Read the model definition and answer for the solid it produces. Units are mm, in the model's axes. A direction names the side the tool comes from. Coordinates: 2 decimals unless noted, no trailing zeros. Loops run counter-clockwise (first coordinate to the right, second up) from the corner with the lowest first, then second, coordinate; pieces in that order, holes last. Notation, with made-up numbers: (-12, 51) - (6, 51) arc R19 ccw to (6, 59) - close; hole circle Ø1 at (-32.75, -1). An arc over 180 degrees is marked (long way). Use one line per item in the form item = value. Start each with the question number.
1) A cutting plane is placed at D-D (y = -17.25). Give the vertices of the cut face in (x, z) (1 decimal).
2) A cutting plane is placed at B-B (x = -19.5). Give the vertices of the cut face in (y, z) (3 decimals).
3) The mould has two halves that part along Z. Classify faces 1 (the face through (3, -20.955, -34)), 2 (the face through (40.42, -14, 0)), 3 (the face through (6.616, -14, 35)), 4 (the face through (-20.493, -14.087, -34.841)): released by +Z, released by -Z, zero draft, split by the parting line, or undercut.
4) A cutting plane is placed at A-A (y = -25.5). Give the vertices of the cut face in (x, z), and give its area (3 significant figures).
5) Which of the six approach directions +Z, -Z, +X, -X, +Y, -Y give full straight-line access (tool end or side, diameter ignored) to faces 5 (the face through (-3, -7.62, -34)), 6 (the face through (20.493, -14.087, 34.841)), 7 (the face through (-6.616, -14, 35))?
6) Each of these flat-tipped pins is pushed along its axis until it touches: P1, Ø2, axis at x = 28.5, y = -17.5, coming from the -Z side; P2, Ø5.5, axis at y = -16, z = 35.5, coming from the -X side; P3, Ø5.5, axis at y = -14, z = 36, coming from the +X side; P4, Ø2, axis at x = 5, z = -37.5, coming from the +Y side. Where does it stop, or does it pass through?
7) A cutting plane is placed at C-C (z = 30.5). Give the vertices of the cut face in (x, y) (3 decimals), and give its area (3 significant figures).
8) Consider line 1 (X direction, y = -11, z = 0); line 2 (X direction, y = -23.25, z = 0); line 3 (Y direction, x = -18, z = -31) (3 decimals). Determine where each line is inside the solid, lowest interval first.
from build123d import *
from build123d import SkipClean  # not in build123d's __all__

# Parameters (mm, degrees)
F0_R     = 44.45
F1_DEPTH = 38.1
F2_R     = 50.8
F3_DEPTH = 10.16
F4_R     = 50.8
F5_DEPTH = 10.16
F7_DEPTH = 25.4
F8_SCALE = 0.75


with BuildPart() as f1:
    # F0 (on Front) → F1 (new body)
    with BuildSketch(Plane.XZ):
        Polygon((53.8927608775, 31.115), (0, 62.23), (-53.8927608775, 31.115), (-53.8927608775, -31.115), (0, -62.23), (53.8927608775, -31.115), align=None)
        Circle(F0_R, mode=Mode.SUBTRACT)
    extrude(amount=F1_DEPTH)

    # F2 (on face) → F3 (cut)
    with BuildSketch(Plane.XZ.offset(38.1)):
        Circle(F2_R)
    extrude(amount=-F3_DEPTH, mode=Mode.SUBTRACT)

    # F4 (on face) → F5 (cut)
    with BuildSketch(Plane(origin=(0, 0, 0), x_dir=(-1, 0, 0), z_dir=(0, 1, 0))):
        Circle(F4_R)
    extrude(amount=-F5_DEPTH, mode=Mode.SUBTRACT)

    # F6 (on face) → F7 (cut)
    with BuildSketch(Plane(origin=(0, -10.16, 0), x_dir=(-1, 0, 0), z_dir=(0, 1, 0))):
        with BuildLine():
            Line((7.7186614973, 43.7747046214), (8.8213274255, 50.028233853))
            ThreePointArc((8.8213274255, 50.028233853), (0, 50.8), (-8.8213274255, 50.028233853))
            Line((-8.8213274255, 50.028233853), (-7.7186614973, 43.7747046214))
            ThreePointArc((-7.7186614973, 43.7747046214), (0, 44.45), (7.7186614973, 43.7747046214))
        make_face()
        with BuildLine():
            Line((-7.7186614973, 43.7747046214), (-8.8213274255, 50.028233853))
            Line((-8.8213274255, 50.028233853), (-8.8213274255, 43.5658889781))
            ThreePointArc((-8.8213274255, 43.5658889781), (-8.2706535041, 43.6737769218), (-7.7186614973, 43.7747046214))
        make_face()
        with BuildLine():
            Line((8.8213274255, 43.5658889781), (8.8213274255, 50.028233853))
            Line((8.8213274255, 50.028233853), (7.7186614973, 43.7747046214))
            ThreePointArc((7.7186614973, 43.7747046214), (8.2706535041, 43.6737769218), (8.8213274255, 43.5658889781))
        make_face()
    with SkipClean():  # cleaning this boolean's faces spoils the solid; the shape is the same uncleaned
        extrude(amount=-F7_DEPTH, mode=Mode.SUBTRACT)


with BuildPart() as f1_1:
    # F8: moved
    add(f1.part.scale(F8_SCALE), clean=False)


solid = f1_1.part
Found:
q1.outline = (-40.4, -23.3) - (0, -46.7) - (40.4, -23.3) - (40.4, 23.3) - (0, 46.7) - (-40.4, 23.3) - close; hole (-6.6, 32.7) arc R33.3 ccw (long way) to (6.6, 32.7) - (6.6, 37.5) arc R38.1 ccw to (-6.6, 37.5) - close
q2.outline = (-28.575, -35.414) - (0, -35.414) - (0, -32.732) - (-7.62, -32.732) - (-7.62, -27.04) - (-20.955, -27.04) - (-20.955, -32.732) - (-28.575, -32.732) - close; (-28.575, 32.732) - (-20.955, 32.732) - (-20.955, 27.04) - (-7.62, 27.04) - (-7.62, 32.732) - (0, 32.732) - (0, 35.414) - (-28.575, 35.414) - close
q3.face_1 = undercut
q3.face_2 = zero draft
q3.face_3 = undercut
q3.face_4 = released by -Z
q4.outline = (-40.42, -23.34) - (0, -46.67) - (40.42, -23.34) - (40.42, 23.34) - (0, 46.67) - (-40.42, 23.34) - close; hole circle Ø76.2 at (0, 0)
q4.area = 1,100 mm^2
q5.face_5 = +Y
q5.face_6 = +Z, +X, +Y, -Y
q5.face_7 = +Y, -Y
q6.P1 = -30.8
q6.P2 = -24.11
q6.P3 = 23.25
q6.P4 = 0
q7.outline = (-28.012, -28.575) - (-22.833, -28.575) - (-22.833, -20.955) - (-13.459, -20.955) - (-13.459, -7.62) - (-22.833, -7.62) - (-22.833, 0) - (-28.012, 0) - close; (13.459, -20.955) - (22.833, -20.955) - (22.833, -28.575) - (28.012, -28.575) - (28.012, 0) - (22.833, 0) - (22.833, -7.62) - (13.459, -7.62) - close
q7.area = 546 mm^2
q8.line_1 = -40.42 to -33.34, 33.34 to 40.42
q8.line_2 = -40.42 to -38.1, 38.1 to 40.42
q8.line_3 = -20.955 to -7.62
